```python
from build123d import *

# Parameters (mm, degrees)
F1_DEPTH  = 8.75
F3_DEPTH  = 2.5
F4_R      = 1
F6_DEPTH  = 6
F8_DEPTH  = 2.5
F9_R      = 1
F11_W     = 9.5
F11_H     = 36
F12_DEPTH = 4
F13_R     = 1


# Not quite as in the source:
# - a feature of the source that left no trace in its solid (it failed there, or was rolled back) is left out
# - a pattern or mirror of a feature is missing from the dataset's text; its kind, count and spacing are read off the source's solid


with BuildPart() as f1:
    # F0 (on Right) → F1 (new body)
    with BuildSketch(Plane.YZ):
        Polygon((3, -5), (3, 0), (47, 0), (49.3, 2.2), (53, 2.2), (54, 3.2), (53.6, 5.45), (52, 6.2), (50, 4.7), (47.5, 4.5), (47, 6), (-0.5, 6), (-0.5, 0), (0, 0), (0, -5), align=None)
    extrude(amount=-F1_DEPTH)

    # F1_copies: F1 across plane


with BuildPart() as f1_1:
    add(f1.part)
    add(f1.part.mirror(Plane(origin=(-8.75, 0, 0), x_dir=(0, 0, -1), z_dir=(-1, 0, 0))))

    # F2 (on face) → F3 (cut)
    with BuildSketch(Plane.YZ):
        Polygon((6, 1.6765981284), (10.3234018716, 6), (6, 6), (6, 5), (1, 0), (-4.5781525858, 0), (-4.5781525858, -7.2408299893), (8, -7.2408299893), (8, 0), (6, 0), align=None)
        Polygon((41, 0), (39, 0), (39, 1.6765981284), (43.3234018716, 6), (39, 6), (39, 5), (34, 0), (28.4218474142, 0), (28.4218474142, -7.2408299893), (41, -7.2408299893), align=None)
        Polygon((74, 0), (72, 0), (72, 1.6765981284), (76.3234018716, 6), (72, 6), (72, 5), (67, 0), (61.4218474142, 0), (61.4218474142, -7.2408299893), (74, -7.2408299893), align=None)
    f3 = extrude(amount=-F3_DEPTH, mode=Mode.SUBTRACT)

    # F3_copies: F3 across plane
    add(f3.mirror(Plane(origin=(-8.75, 0, 0), x_dir=(0, 0, -1), z_dir=(-1, 0, 0))), mode=Mode.SUBTRACT)

    # F4
    f4_edges = [f1_1.edges().sort_by_distance(p)[0] for p in [
        (-8.75, 47, 6),
    ]]
    fillet(f4_edges, radius=F4_R)

    # F5 (on face) → F6 (join, through all)
    with BuildSketch(Plane.XY.offset(6)):
        with BuildLine():
            Line((-6.75, -0.5), (-8.75, -0.5))
            Line((-8.75, -0.5), (-8.75, -5.5))
            Line((-8.75, -5.5), (-6.75, -5.5))
            Line((-6.75, -5.5), (-5.6642135624, -4.4142135624))
            Line((-5.6642135624, -4.4142135624), (5.6286796564, -15.7071067812))
            ThreePointArc((5.6286796564, -15.7071067812), (7.0428932188, -15.7071067812), (7.0428932188, -14.2928932188))
            Line((7.0428932188, -14.2928932188), (-6.75, -0.5))
        make_face()
    f6 = extrude(amount=-F6_DEPTH)

    # F6_copies: F6 across plane
    add(f6.mirror(Plane(origin=(-8.75, 0, 0), x_dir=(0, 0, -1), z_dir=(-1, 0, 0))))

    # F7 (on face) → F8 (cut)
    with BuildSketch(Plane.YZ):
        Polygon((46.5, 7.9169040546), (46.5, 6), (47, 0), (57.128790766, 0), (57.128790766, 7.9169040546), align=None)
    f8 = extrude(amount=-F8_DEPTH, mode=Mode.SUBTRACT)

    # F8_copies: F8 across plane
    add(f8.mirror(Plane(origin=(-8.75, 0, 0), x_dir=(0, 0, -1), z_dir=(-1, 0, 0))), mode=Mode.SUBTRACT)

    # F9
    f9_edges = [f1_1.edges().sort_by_distance(p)[0] for p in [
        (-5.664214, -4.414214, 3),
        (-8.75, 3, 0),
        (-10.75, -0.5, 3),
        (-11.835786, -4.414214, 3),
        (-6.75, -0.5, 3),
    ]]
    fillet(f9_edges, radius=F9_R)

    # F11 (on face) → F12 (cut)
    with BuildSketch(Plane(origin=(0, 0, 0), x_dir=(1, 0, 0), z_dir=(0, 0, -1))):
        with Locations((-8.75, -25)):
            Rectangle(F11_W, F11_H)
    extrude(amount=-F12_DEPTH, mode=Mode.SUBTRACT)

    # F13
    f13_edges = [f1_1.edges().sort_by_distance(p)[0] for p in [
        (-13.5, 7, 2),
        (-4, 7, 2),
        (-13.5, 43, 2),
        (-4, 43, 2),
    ]]
    fillet(f13_edges, radius=F13_R)


solid = f1_1.part
```
Geometry: final body of the model. Coordinates: model frame, mm. A direction names the side the tool comes from. Give positions to 0.01 mm unless a question says otherwise; leave off trailing zeros. Loops run counter-clockwise (first coordinate to the right, second up) from the corner with the lowest first, then second, coordinate; pieces in that order, holes last. Notation, with made-up numbers: (86.25, -38.75) -> (98.25, -38.75) arc R16 ccw to (98.25, -33.75) -> close; hole circle Ø9 at (25.5, 27.5). An arc over 180 degrees is marked (long way). Return JSON: item names as keys, results as strings.
Item 1: Mould query, pull axis Y, two halves, no side actions, for faces 6 (the flat face through (-16, 6, 1)), 7 (the flat face through (-16.267, 46.748, 3.029)), 8 (the flat face through (0, 2, 4)). Classes: released by +Y, released by -Y, zero draft, split by the parting line, or undercut.
Filled in:
{"face 6": "undercut", "face 7": "released by +Y", "face 8": "zero draft"}
Item 2: Section B-B, the plane y = -15. Output: boundary loops of the cut face in (x, z), plus the area to 3 significant figures.
Filled in:
{"outline": "(-24.84, 0) -> (-22.42, 0) -> (-22.42, 6) -> (-24.84, 6) -> close; (4.92, 0) -> (7.34, 0) -> (7.34, 6) -> (4.92, 6) -> close", "area": "29.0 mm^2"}
Item 3: Line query: line 1 (X direction, y = 39, z = 3.25); line 2 (Y direction, x = -0.5, z = 4.75); line 3 (X direction, y = 30.5, z = 2.75). Output: solid intervals per line, ascending.
Filled in:
{"line 1": "-15 to -13.5, -4 to -2.5", "line 2": "-9.58 to -6.75, -0.5 to 5.75, 9.07 to 38.75, 42.07 to 46.6", "line 3": "-17.5 to -13.5, -4 to 0"}
Item 4: Pin query (flat end, axial travel): P1, Ø3, axis at x = -3.5, z = -0.5, coming from the +Y side; P2, Ø1, axis at y = 23, z = 4.5, coming from the +X side; P3, Ø6, axis at x = -6.5, z = -2, coming from the -Y side. Return the tip coordinate at first contact, or that it passes through.
Filled in:
{"P1": "y = 48.05", "P2": "x = 0", "P3": "y = -5.81"}
Item 5: Section A-A, the plane x = -10. Output: boundary loops of the cut face in (y, z).
Filled in:
{"outline": "(-5.5, 0) -> (0, 0) -> (0, -5) -> (3, -5) -> (3, -1) arc R1 cw to (4, 0) -> (7, 0) -> (7, 4) -> (43, 4) -> (43, 0) -> (47, 0) -> (49.3, 2.2) -> (53, 2.2) -> (54, 3.2) -> (53.6, 5.45) -> (52, 6.2) -> (50, 4.7) -> (47.5, 4.5) -> (47.23, 5.32) arc R1 ccw to (46.28, 6) -> (-5.5, 6) -> close"}
Item 6: Section D-D, the plane z = -4. Output: boundary loops of the cut face in (x, y).
Filled in:
{"outline": "(-15, 0) -> (-2.5, 0) -> (-2.5, 3) -> (-15, 3) -> close"}
Item 7: Section C-C, the plane y = 14. Output: boundary loops of the cut face in (x, z), plus the area to 3 significant figures.
Filled in:
{"outline": "(-17.5, 0) -> (-13.5, 0) -> (-13.5, 4) -> (-4, 4) -> (-4, 0) -> (0, 0) -> (0, 6) -> (-17.5, 6) -> close", "area": "67.0 mm^2"}
Item 8: Access query for faces 1 (the flat face through (-9, 43, 2)), 2 (the flat face through (1.08, -8.33, 3.04)), 3 (the flat face through (-17.5, 2, 4)), 4 (the flat face through (-1.232, 46.748, 3.029)), 5 (the flat face through (-9, 3, -3)). Directions: +Z, -Z, +X, -X, +Y, -Y. A direction counts if a zero-diameter tool reaches every point of the face in a straight line with its end or side. Return the directions, or none.
Filled in:
{"face 1": "-Z", "face 2": "+Z, -Z, +X", "face 3": "+Z, -Z, -X, +Y", "face 4": "+Z, +X, +Y", "face 5": "-Z, +X, -X, +Y"}
